from build123d import *


with BuildPart() as part:
    # Esquisse1 → Révolution1789 (revolve)
    with BuildSketch(Plane.XY, mode=Mode.PRIVATE) as r_volution1789_sk:
        Polygon((0, 18), (-3.5, 18), (-3.5, 15), (-4.5, 15), (-4.5, 15.5), (-8, 15.5), (-8.5, 15), (-8.5, 12), (-5.75, 12), (-5, 11.25), (-5, 5.75), (-5.75, 5), (-8.5, 5), (-8.5, 2.5), (-3, 2.5), (-3, 6), (0, 6), align=None)
    revolve(r_volution1789_sk.sketch.rotate(Axis((0, 0, 0), (-1, 0, 0)), 90), axis=Axis((0, 0, 0), (-1, 0, 0)))


solid = part.part
For this review, take the finished solid that the model builds, in its own axes (mm). A direction names the side the tool comes from. Round coordinates to 2 decimals unless told otherwise and drop trailing zeros. Put each result on its own line as item: value.
Q1. Mouldability with a two-part tool opening along Z and no side actions: class faces 1 (the cylindrical face through (-5.7, -0.1, 2.5)), 2 (the cylindrical face through (-1.774, -12.165, 13.267)), 3 (the flat face through (-8.5, 2, -2)) as pulls with the +Z half, pulls with the -Z half, needs draft (parallel to the pull), parting line crosses it, or undercut.
Check result:
face 1: undercut
face 2: parting line crosses it
face 3: needs draft
Q2. For probe 1 along Y at (x, z) = (-6.3, 0); probe 2 along Y at (x, z) = (-1.75, 0); probe 3 along Y at (x, z) = (-4.6, 0), list the stretches that pass through material, from the lowest coordinate up. Write a range as [from, to].
Check result:
probe 1: [-15.5, -12], [-5, -2.5], [2.5, 5], [12, 15.5]
probe 2: [-18, -6], [6, 18]
probe 3: [-15.5, -2.5], [2.5, 15.5]
Q3. Machinability: for faces 4 (the cylindrical face through (-1.479, -1.802, -5.723)), 5 (the cylindrical face through (-7, 0, 5)), 6 (the cylindrical face through (-4.01, -12.65, -8.06)), which of the approach directions +Z, -Z, +X, -X, +Y, -Y give a long, thin tool a straight path to every point of the face, cutting with its end or side? Answer none if there is none.
Check result:
face 4: +X
face 5: -X
face 6: none
Q4. Insertion check: pin 1 Ø5 at (x, z) = (-6.5, -7) entering from -Y; pin 2 Ø1.5 at (x, y) = (-3.5, -2.5) entering from -Z; pin 3 Ø2 at (x, z) = (-2.5, 7) entering from -Y. Each pin has a flat end and moves straight along its axis. Give the tip position at first contact, or say it passes through.
Check result:
pin 1: y = -14.83
pin 2: z = -17.91
pin 3: y = -16.97
